from build123d import *

# Parameters (mm, degrees)
SKETCH1_W           = 880
SKETCH1_H           = 580
BOSS_EXTRUDE1_DEPTH = 35
SKETCH2_R           = 20
CUT_EXTRUDE1_DEPTH  = 202
SKETCH3_R           = 25
CUT_EXTRUDE2_DEPTH  = 10


with BuildPart() as part:
    # Sketch1 → Boss-Extrude1 (new body)
    with BuildSketch(Plane(origin=(0, 0, 0), x_dir=(1, 0, 0), z_dir=(0, 1, 0))):
        Rectangle(SKETCH1_W, SKETCH1_H)
    extrude(amount=BOSS_EXTRUDE1_DEPTH)

    # Sketch2 → Cut-Extrude1 (cut)
    with BuildSketch(Plane.XZ):
        with Locations(Location((-340, 140, 0), (0, 0, 270))):
            Circle(SKETCH2_R)
        with Locations(Location((340, 140, 0), (0, 0, 270))):
            Circle(SKETCH2_R)
        with Locations(Location((340, -140, 0), (0, 0, 90))):
            Circle(SKETCH2_R)
        with Locations(Location((-340, -140, 0), (0, 0, 90))):
            Circle(SKETCH2_R)
    extrude(amount=-CUT_EXTRUDE1_DEPTH, mode=Mode.SUBTRACT)

    # Sketch3 → Cut-Extrude2 (cut)
    with BuildSketch(Plane.XZ):
        with Locations(Location((-340, 140, 0), (0, 0, 270))):
            Circle(SKETCH3_R)
        with Locations(Location((340, 140, 0), (0, 0, 270))):
            Circle(SKETCH3_R)
        with Locations(Location((340, -140, 0), (0, 0, 270))):
            Circle(SKETCH3_R)
        with Locations(Location((-340, -140, 0), (0, 0, 270))):
            Circle(SKETCH3_R)
    extrude(amount=-CUT_EXTRUDE2_DEPTH, mode=Mode.SUBTRACT)


solid = part.part
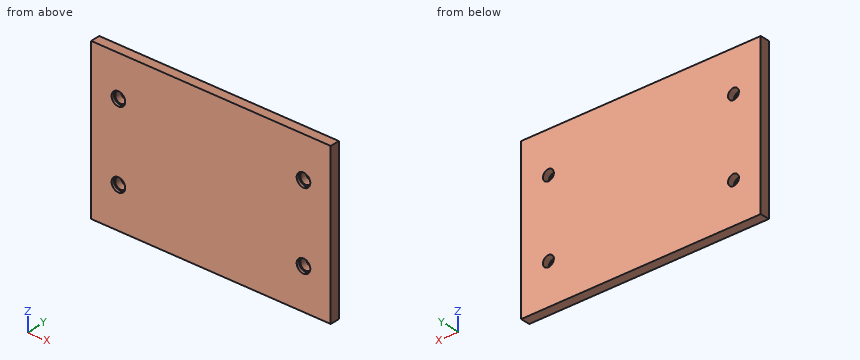
Build history of the part. All positions in model axes, mm. Coordinates: 2 decimals unless noted, no trailing zeros. Order: outer loops, then holes, each group sorted by start corner. A loop starts at its lowest first (then second) coordinate and runs counter-clockwise, first axis right, second up. Notation, with made-up numbers: M 32,52 L 50,52 A29 cw 50,77 Z; hole C -24.5,29 d1. An arc over 180 degrees is marked long. One line per question, with ' | ' between items. Start each with the question number.
Q1. Saw through at B-B (x = 340). List the corners of the cut face in (y, z), then the cut area to 3 significant figures.
Q2. Saw through at A-A (z = 140). List the corners of the cut face in (x, y).
Q3. Probe L1, parallel to X at y = 6.25, z = 140; L2, parallel to X at y = 25, z = -140. List the from-to ranges inside material, lowest first. Write a range as from..to.
Q4. Flat gauge pin, fed straight in: pin 1 Ø1.5 at (x, z) = (274, -56) entering from -Y. Where does the tip first touch, or does it go through?
Check values:
1) outline: M 0,-290 L 35,-290 L 35,-160 L 10,-160 L 10,-165 L 0,-165 Z; M 0,-115 L 10,-115 L 10,-120 L 35,-120 L 35,120 L 10,120 L 10,115 L 0,115 Z; M 0,165 L 10,165 L 10,160 L 35,160 L 35,290 L 0,290 Z | area: 17,300 mm2
2) outline: M -440,0 L -365,0 L -365,10 L -360,10 L -360,35 L -440,35 Z; M -320,10 L -315,10 L -315,0 L 315,0 L 315,10 L 320,10 L 320,35 L -320,35 Z; M 360,10 L 365,10 L 365,0 L 440,0 L 440,35 L 360,35 Z
3) L1: x = -440..-365, -315..315, 365..440 | L2: x = -440..-360, -320..320, 360..440
4) pin 1: stops at y = 0
